```python
from build123d import *

# Parameters (mm, degrees)
BOSS_EXTRUDE1_DEPTH  = 25.4
CHAMFER1_SIZE        = 0.79375
SKETCH2_R            = 0.889
CUT_EXTRUDE1_DEPTH   = 27.940768363
M2_CLEARANCE_HOLE1_D = 2.4
FILLET1_RADIUS       = 3.175
FILLET1_LENGTH       = 25.4
FILLET2_R            = 4.7625
FILLET3_R            = 1.5875


with BuildPart() as part:
    # Sketch1 → Boss-Extrude1 (new body)
    with BuildSketch(Plane.XY):
        Polygon((0, 0), (0, 5.55625), (-6.35, 5.55625), (-6.35, -6.35), (4.7625, -6.35), (4.7625, 0), align=None)
    extrude(amount=BOSS_EXTRUDE1_DEPTH)

    # Chamfer1
    chamfer1_edges = [part.edges().sort_by_distance(p)[0] for p in [
        (0, 0, 12.7),
    ]]
    chamfer(chamfer1_edges, length=CHAMFER1_SIZE)

    # Sketch2 → Cut-Extrude1 (cut, through all)
    with BuildSketch(Plane.XY.offset(25.4)):
        with Locations((-0.79375, -2.90315)):
            Circle(SKETCH2_R)
    extrude(amount=-CUT_EXTRUDE1_DEPTH, mode=Mode.SUBTRACT)

    # M2 Clearance Hole1 (through all)
    with Locations(Plane(origin=(0, 0, 0), x_dir=(0, 0, -1), z_dir=(1, 0, 0))):
        with Locations((-20.7609375, 2.5), (-4.7609375, 2.5)):
            Hole(M2_CLEARANCE_HOLE1_D / 2)

    # Fillet1: full round fillet: the end face becomes a half cylinder, R = half its width
    fillet1_face = Plane((4.7625, -3.175, 12.7), x_dir=(0, 0, 1), z_dir=(1, 0, 0))  # on the end face: x along it, z out of the body
    fillet1_slab = fillet1_face.offset(-FILLET1_RADIUS / 2) * Box(FILLET1_LENGTH, 2 * FILLET1_RADIUS, FILLET1_RADIUS, mode=Mode.PRIVATE)  # the body's end, R deep
    fillet1_round = Plane((1.5875, -3.175, 12.7), x_dir=(1, 0, 0), z_dir=(0, 0, 1)) * Cylinder(FILLET1_RADIUS, FILLET1_LENGTH, mode=Mode.PRIVATE)  # its axis R under the face
    add(fillet1_slab - fillet1_round, mode=Mode.SUBTRACT)

    # Fillet2
    fillet2_edges = [part.edges().sort_by_distance(p)[0] for p in [
        (-6.35, -6.35, 12.7),
    ]]
    fillet(fillet2_edges, radius=FILLET2_R)

    # Fillet3
    fillet3_edges = [part.edges().sort_by_distance(p)[0] for p in [
        (-3.175, 5.55625, 25.4),
        (-3.175, 5.55625, 0),
    ]]
    fillet(fillet3_edges, radius=FILLET3_R)


solid = part.part
```
The listing builds one solid part. Answer for the finished solid, in the listing's coordinates (mm). A direction names the side the tool comes from. Coordinates: 2 decimals unless noted, no trailing zeros. Write each loop counter-clockwise with the first axis right and the second up, starting at its lowest first coordinate (ties: lowest second). Pieces come first, ordered by that corner, then holes. Notation, with made-up numbers: (58, -34.5) -> (92, -34.5) arc R15 ccw to (92, -30.5) -> close; hole circle Ø11 at (12.5, -18). An arc over 180 degrees is marked (long way). Write each question's results on one line, items separated by ' | '. Start each with the question number.
1) A cutting plane is placed at D-D (x = -5.25). Determine the outline of the cut face in (y, z) (1 decimal).
2) A cutting plane is placed at B-B (x = -1.25). Count the separate pieces of the cut face and the enclosed holes in it, then the cut area to 3 significant figures.
3) Flat-ended cylindrical pins translate along their axes: pin 1 Ø2.5 at (y, z) = (3.5, 16) entering from +X; pin 2 Ø2 at (y, z) = (2.5, 20.76) entering from +X; pin 3 Ø3 at (x, z) = (-2.5, 5) entering from -Y. Find the tip coordinate at first contact, or state that the pin passes through.
4) Straight lines are drawn through the part: probe 1 along Z at (x, y) = (-1, 3.25); probe 2 along Y at (x, z) = (1, 16); probe 3 along X at (y, z) = (-2.5, 16.5). For each, find the intervals that lie inside material, in ascending order.
5) For a pull along Z with two mould halves and no side action, classify faces 1 (the cylindrical face through (-3.22, 2.55, 3.56)), 2 (the cylindrical face through (-3.219, 5.079, 0.453)), 3 (the cylindrical face through (-4.99, -4.92, 12.88)), 4 (the cylindrical face through (-3.22, 2.55, 19.56)) as +Z half, -Z half, draft (parallel to the pull), parting line (faces both ways), or undercut.
6) A tool of negligible diameter and unlimited length cuts with its end or side. For faces 5 (the flat face through (0, 3, 13)), 6 (the flat face through (-2, -1, 0)), from which of +Z, -Z, +X, -X, +Y, -Y can it reach the whole face along a straight path? Write none if from no direction.
7) A cutting plane is placed at A-A (y = 2.5). Determine the outline of the cut face in (x, z), then the cut area to 3 significant figures.
Values follow:
1) outline: (-4.6, 0) -> (4, 0) arc R1.6 ccw to (5.6, 1.6) -> (5.6, 23.8) arc R1.6 ccw to (4, 25.4) -> (-4.6, 25.4) -> close; hole circle Ø2.4 at (2.5, 4.8); hole circle Ø2.4 at (2.5, 20.8)
2) separate pieces: 2 | enclosed holes: 2 | area: 254 mm²
3) pin 1: x = 0 | pin 2: through | pin 3: y = -6.35
4) probe 1: 0 to 3.82, 5.7 to 19.82, 21.7 to 25.4 | probe 2: -6.35 to 0 | probe 3: -6.26 to -1.59, 0 to 4.69
5) face 1: undercut | face 2: -Z half | face 3: draft | face 4: undercut
6) face 5: +Z, -Z, +X, +Y | face 6: -Z, +X, -X, +Y, -Y
7) outline: (-6.35, 0) -> (0, 0) -> (0, 3.56) -> (-6.35, 3.56) -> close; (-6.35, 5.96) -> (0, 5.96) -> (0, 19.56) -> (-6.35, 19.56) -> close; (-6.35, 21.96) -> (0, 21.96) -> (0, 25.4) -> (-6.35, 25.4) -> close | area: 131 mm²
